from build123d import *

# Parameters (mm, degrees)
F0_W     = 609.6
F0_H     = 1143
F1_DEPTH = 609.6
F2_W     = 508
F2_H     = 1092.2
F3_DEPTH = 6.35
F4_R     = 25.4
F5_DEPTH = 25.4


with BuildPart() as f1:
    # F0 (on Right) → F1 (new body)
    with BuildSketch(Plane.YZ):
        with Locations((-76.00952, 7.364793)):
            Rectangle(F0_W, F0_H)
    extrude(amount=F1_DEPTH)

    # F2 (on face) → F3 (join)
    with BuildSketch(Plane.YZ.offset(609.6)):
        with Locations((-76.00952, -18.035207)):
            Rectangle(F2_W, F2_H)
    extrude(amount=F3_DEPTH)

    # F4 (on face) → F5 (join)
    with BuildSketch(Plane.YZ.offset(615.95)):
        with Locations((127.19048, 0)):
            Circle(F4_R)
    extrude(amount=F5_DEPTH)


solid = f1.part
Source: CAD feature listing. Evaluate the final solid. Frame: model axes, mm. A direction names the side the tool comes from. Give positions to 0.01 mm unless a question says otherwise; leave off trailing zeros. Order: outer loops, then holes, each group sorted by start corner. A loop starts at its lowest first (then second) coordinate and runs counter-clockwise, first axis right, second up. Notation, with made-up numbers: (1, -12) -> (60, -12) arc R19 cw to (60, 21) -> close; hole circle Ø4 at (52, 34.5). An arc over 180 degrees is marked (long way). Write item = value, one per line.
Q1. Cut plane B-B, the plane y = -318. Output: boundary loops of the cut face in (x, z), and give its area (3 significant figures).
Data:
outline = (0, -564.14) -> (615.95, -564.14) -> (615.95, 528.06) -> (609.6, 528.06) -> (609.6, 578.86) -> (0, 578.86) -> close
area = 704,000 mm^2
Q2. Cut plane A-A, the plane z = 480.5. Output: boundary loops of the cut face in (x, y), and give its area (3 significant figures).
Data:
outline = (0, -380.81) -> (609.6, -380.81) -> (609.6, -330.01) -> (615.95, -330.01) -> (615.95, 177.99) -> (609.6, 177.99) -> (609.6, 228.79) -> (0, 228.79) -> close
area = 375,000 mm^2
Q3. Material intervals for line 1 (X direction, y = 85.5, z = -106); line 2 (X direction, y = -333, z = 359), sorted ascending. Write a range as from..to.
Data:
line_1 = 0..615.95
line_2 = 0..609.6
Q4. Cut plane C-C, the plane z = 0. Output: boundary loops of the cut face in (x, y).
Data:
outline = (0, -380.81) -> (609.6, -380.81) -> (609.6, -330.01) -> (615.95, -330.01) -> (615.95, 101.79) -> (641.35, 101.79) -> (641.35, 152.59) -> (615.95, 152.59) -> (615.95, 177.99) -> (609.6, 177.99) -> (609.6, 228.79) -> (0, 228.79) -> close
Q5. Set-up query: faces 1 (the face through (0, -80, 15)), 2 (the face through (628.472, 101.815, 1.117)). Return all of +Z, -Z, +X, -X, +Y, -Y with unobstructed straight access to the full face (end or side cutting, diameter ignored); none if empty.
Data:
face_1 = +Z, -Z, -X, +Y, -Y
face_2 = +X
Q6. Pin query (flat end, axial travel): pin 1 (5 mm diameter, centred on x = 612.5, z = -59.5, fed in from -Y); pin 2 (12 mm diameter, centred on y = -50.5, z = 49, fed in from +X); pin 3 (5 mm diameter, centred on x = 614, z = 137, fed in from +Y). Return the tip coordinate at first contact, or that it passes through.
Data:
pin_1 = -330.01
pin_2 = 615.95
pin_3 = 177.99
